Geometry check sheet. Reference: the model listing, model coordinates, mm. Coordinates: 2 decimals unless noted, no trailing zeros. Loops run counter-clockwise (first coordinate to the right, second up) from the corner with the lowest first, then second, coordinate; pieces in that order, holes last. Notation, with made-up numbers: (56, 77.25) - (106, 77.25) arc R11 ccw to (106, 97.25) - close; hole circle Ø5 at (16, -37). An arc over 180 degrees is marked (long way). Write item = value, one per line. Start each with the question number.
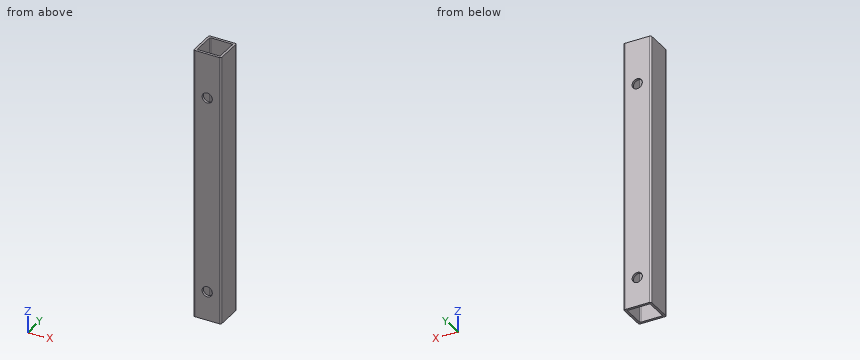
from build123d import *

# Parameters (mm, degrees)
DODANIE_WYCI_GNI_CIE1_DEPTH = 345
SZKIC2_R                    = 6.5
WYTNIJ_WYCI_GNI_CIE1_DEPTH  = 345


with BuildPart() as part:
    # Szkic1 → Dodanie-wyciągnięcie1 (new body)
    with BuildSketch(Plane.XY):
        with BuildLine():
            Line((2, 0), (33, 0))
            ThreePointArc((33, 0), (34.414213562, 0.585786438), (35, 2))
            Line((35, 2), (35, 33))
            ThreePointArc((35, 33), (34.414213562, 34.414213562), (33, 35))
            Line((33, 35), (2, 35))
            ThreePointArc((2, 35), (0.585786438, 34.414213562), (0, 33))
            Line((0, 33), (0, 2))
            ThreePointArc((0, 2), (0.585786438, 0.585786438), (2, 0))
        make_face()
        with BuildLine():
            Line((4, 3), (31, 3))
            ThreePointArc((31, 3), (31.707106781, 3.292893219), (32, 4))
            Line((32, 4), (32, 31))
            ThreePointArc((32, 31), (31.707106781, 31.707106781), (31, 32))
            Line((31, 32), (4, 32))
            ThreePointArc((4, 32), (3.292893219, 31.707106781), (3, 31))
            Line((3, 31), (3, 4))
            ThreePointArc((3, 4), (3.292893219, 3.292893219), (4, 3))
        make_face(mode=Mode.SUBTRACT)
    extrude(amount=DODANIE_WYCI_GNI_CIE1_DEPTH)

    # Szkic2 → Wytnij-wyciągnięcie1 (cut)
    with BuildSketch(Plane(origin=(0, 35, 0), x_dir=(1, 0, 0), z_dir=(0, 1, 0))):
        with Locations(Location((17.5, -288, 0), (0, 0, 270))):
            Circle(SZKIC2_R)
        with Locations(Location((17.5, -37, 0), (0, 0, 270))):
            Circle(SZKIC2_R)
    extrude(amount=-WYTNIJ_WYCI_GNI_CIE1_DEPTH, mode=Mode.SUBTRACT)


solid = part.part
(1) Sectioned sample at A-A on z = 37. Enter the section's corners in (x, y).
(2) Sectioned sample at B-B on y = 12. Enter the section's corners in (x, z), plus the area to 3 significant figures.
(3) Sectioned sample at C-C on x = 17.5. Enter the section's corners in (y, z).
(4) Scan lines: line 1 (Z direction, x = 17, y = 33); line 2 (X direction, y = 13, z = 315). Record each from-to range of solid material in increasing order.
(5) Sectioned sample at D-D on z = 116. Enter the section's corners in (x, y).
Working result:
q1.outline = (0, 2) arc R2 ccw to (2, 0) - (11, 0) - (11, 3) - (4, 3) arc R1 cw to (3, 4) - (3, 31) arc R1 cw to (4, 32) - (11, 32) - (11, 35) - (2, 35) arc R2 ccw to (0, 33) - close; (24, 0) - (33, 0) arc R2 ccw to (35, 2) - (35, 33) arc R2 ccw to (33, 35) - (24, 35) - (24, 32) - (31, 32) arc R1 cw to (32, 31) - (32, 4) arc R1 cw to (31, 3) - (24, 3) - close
q2.outline = (0, 0) - (3, 0) - (3, 345) - (0, 345) - close; (32, 0) - (35, 0) - (35, 345) - (32, 345) - close
q2.area = 2,070 mm2
q3.outline = (0, 0) - (3, 0) - (3, 30.5) - (0, 30.5) - close; (0, 43.5) - (3, 43.5) - (3, 281.5) - (0, 281.5) - close; (0, 294.5) - (3, 294.5) - (3, 345) - (0, 345) - close; (32, 0) - (35, 0) - (35, 30.5) - (32, 30.5) - close; (32, 43.5) - (35, 43.5) - (35, 281.5) - (32, 281.5) - close; (32, 294.5) - (35, 294.5) - (35, 345) - (32, 345) - close
q4.line_1 = 0 to 30.52, 43.48 to 281.52, 294.48 to 345
q4.line_2 = 0 to 3, 32 to 35
q5.outline = (0, 2) arc R2 ccw to (2, 0) - (33, 0) arc R2 ccw to (35, 2) - (35, 33) arc R2 ccw to (33, 35) - (2, 35) arc R2 ccw to (0, 33) - close; hole (3, 4) arc R1 ccw to (4, 3) - (31, 3) arc R1 ccw to (32, 4) - (32, 31) arc R1 ccw to (31, 32) - (4, 32) arc R1 ccw to (3, 31) - close
